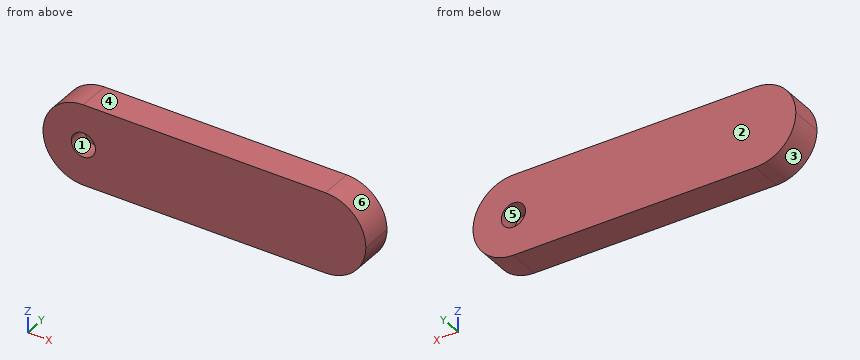
```python
from build123d import *

# Parameters (mm, degrees)
ESBO_O2_W                = 400
ESBO_O2_H                = 100
RESSALTO_EXTRUS_O1_DEPTH = 40
FILETE1_R                = 50
ESBO_O5_R                = 15
CORTE_EXTRUS_O1_DEPTH    = 25
ESBO_O3_R                = 15
CORTE_EXTRUS_O2_DEPTH    = 25


with BuildPart() as part:
    # Esboço2 → Ressalto-extrusão1 (new body)
    with BuildSketch(Plane(origin=(0, 0, 0), x_dir=(1, 0, 0), z_dir=(0, 1, 0))):
        Rectangle(ESBO_O2_W, ESBO_O2_H)
    extrude(amount=RESSALTO_EXTRUS_O1_DEPTH)

    # Filete1
    filete1_edges = [part.edges().sort_by_distance(p)[0] for p in [
        (-200, 20, -50),
        (-200, 20, 50),
        (200, 20, -50),
        (200, 20, 50),
    ]]
    fillet(filete1_edges, radius=FILETE1_R - 0.0001)  # a hair under: the kernel refuses the full size

    # Esboço5 → Corte-extrusão1 (cut)
    with BuildSketch(Plane.XZ):
        with Locations(Location((-150, 0, 0), (0, 0, 270))):
            Circle(ESBO_O5_R)
    extrude(amount=-CORTE_EXTRUS_O1_DEPTH, mode=Mode.SUBTRACT)

    # Esboço3 → Corte-extrusão2 (cut)
    with BuildSketch(Plane(origin=(0, 40, 0), x_dir=(1, 0, 0), z_dir=(0, 1, 0))):
        with Locations(Location((150, 0, 0), (0, 0, 270))):
            Circle(ESBO_O3_R)
    extrude(amount=-CORTE_EXTRUS_O2_DEPTH, mode=Mode.SUBTRACT)


solid = part.part
```
Geometry check sheet. Reference: the model listing, model coordinates, mm. Face numbers are marked on the shaded views. A direction names the side the tool comes from. Round coordinates to 2 decimals unless told otherwise and drop trailing zeros. Order: outer loops, then holes, each group sorted by start corner. A loop starts at its lowest first (then second) coordinate and runs counter-clockwise, first axis right, second up. Notation, with made-up numbers: M 9,83 L 61,83 A15 cw 61,90 Z; hole C -24,69.25 d9. An arc over 180 degrees is marked long. Write item = value, one per line.
Q1. Set-up check for the marked faces 1 and 2: record each of +Z, -Z, +X, -X, +Y, -Y from which the full face is reachable in a straight line by a thin tool's end or side.
Answer block:
face_1 = -Y
face_2 = +Z, -Z, +X, -X, +Y
Q2. Release check for a two-part mould opening along X. For the marked faces 3, 4, 5 and 6 record: released by +X, released by -X, zero draft, split by the parting line, or undercut.
Answer block:
face_3 = released by -X
face_4 = zero draft
face_5 = undercut
face_6 = released by +X
Q3. Depth check by flat-ended pin: pin 1 Ø9 at (x, z) = (-147.5, 6.5) entering from -Y; pin 2 Ø2 at (y, z) = (28, -7.5) entering from +X; pin 3 Ø2 at (y, z) = (32, -38.5) entering from -X. Enter the tip coordinate at first touch or a pass-through.
Answer block:
pin_1 = 25
pin_2 = 199.58
pin_3 = -183.07
Q4. Section check C-C (z = -23.5). Enter the section's corners in (x, y).
Answer block:
outline = M -194.13,0 L 194.13,0 L 194.13,40 L -194.13,40 Z
Q5. Section check B-B (x = 143.5). Enter the section's corners in (y, z), plus the area to 3 significant figures.
Answer block:
outline = M 0,-50 L 40,-50 L 40,-13.52 L 15,-13.52 L 15,13.52 L 40,13.52 L 40,50 L 0,50 Z
area = 3,320 mm^2
Q6. Scan lines: line 1 (X direction, y = 24.5, z = 0); line 2 (X direction, y = 34, z = 0); line 3 (X direction, y = 22.5, z = 10). Record each from-to range of solid material in increasing order.
Answer block:
line_1 = -200 to -165, -135 to 135, 165 to 200
line_2 = -200 to 135, 165 to 200
line_3 = -198.99 to -161.18, -138.82 to 138.82, 161.18 to 198.99
